Design review of the part shown in the three views and the two pictorial views. Dimensions are in mm from the part's minimum x, y and z. A direction names the side the tool comes from. Coordinates: 2 decimals unless noted, no trailing zeros. Write each loop counter-clockwise with the first axis right and the second up, starting at its lowest first coordinate (ties: lowest second). Pieces come first, ordered by that corner, then holes.
Q1. Take a section at B-B, the plane z = 20. Write out the cut boundary in (x, y), plus the area to 3 significant figures.
Q2. Take a section at A-A, the plane x = 12.5. Write out the cut boundary in (y, z), plus the area to 3 significant figures.
Q3. Take a section at D-D, the plane x = 70. Write out the cut boundary in (y, z), plus the area to 3 significant figures.
Q4. For pin 1 Ø3.5 at (x, y) = (145, 140) entering from +Z; pin 2 Ø8 at (y, z) = (87, 11) entering from -X; pin 3 Ø3 at (y, z) = (141.5, 21.5) entering from +X, all flat-tipped, find the tip position at first contact; note any pin that passes through.
Q5. For L1, parallel to Y at x = 5, z = 3.5; L2, parallel to Y at x = 62.5, z = 21.5; L3, parallel to Y at x = 39, z = 21.75, list the stretches that pass through material, from the lowest coordinate up.
Q6. Take a section at C-C, the plane y = 105. Write out the cut boundary in (x, z), plus the area to 4 significant figures.
Q7. The part is to be moulded in two halves that separate along Y. For the marked faces 3, 4 and 5, say which applies: released by +Y, released by -Y, zero draft, split by the parting line, or undercut.
Q8. For the marked faces 1 and 2, list the 3-axis set-ups (+Z, -Z, +X, -X, +Y, -Y) from which the entire face can be reached by the end or side of a thin tool; tool diameter is ignored.
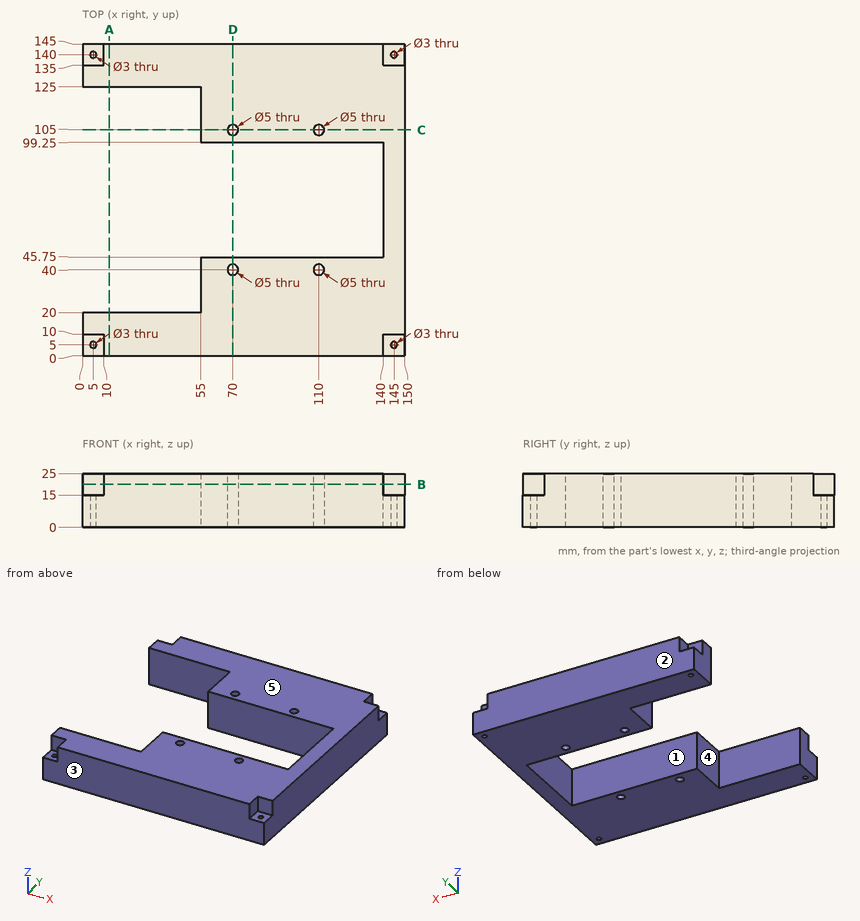
Responses:
1. outline: (0, 10) - (10, 10) - (10, 0) - (140, 0) - (140, 10) - (150, 10) - (150, 135) - (140, 135) - (140, 145) - (10, 145) - (10, 135) - (0, 135) - (0, 125) - (55, 125) - (55, 99.25) - (140, 99.25) - (140, 45.75) - (55, 45.75) - (55, 20) - (0, 20) - close; hole circle Ø5 at (70, 40); hole circle Ø5 at (70, 105); hole circle Ø5 at (110, 40); hole circle Ø5 at (110, 105)
1. area: 10,900 mm2
2. outline: (0, 0) - (20, 0) - (20, 25) - (0, 25) - close; (125, 0) - (145, 0) - (145, 25) - (125, 25) - close
2. area: 1,000 mm2
3. outline: (0, 0) - (37.5, 0) - (37.5, 25) - (0, 25) - close; (42.5, 0) - (45.75, 0) - (45.75, 25) - (42.5, 25) - close; (99.25, 0) - (102.5, 0) - (102.5, 25) - (99.25, 25) - close; (107.5, 0) - (145, 0) - (145, 25) - (107.5, 25) - close
3. area: 2,040 mm2
4. pin 1: stops at z = 15
4. pin 2: stops at x = 140
4. pin 3: stops at x = 140
5. L1: y = 0 to 3.5, 6.5 to 20, 125 to 138.5, 141.5 to 145
5. L2: y = 0 to 45.75, 99.25 to 145
5. L3: y = 0 to 20, 125 to 145
6. outline: (55, 0) - (67.5, 0) - (67.5, 25) - (55, 25) - close; (72.5, 0) - (107.5, 0) - (107.5, 25) - (72.5, 25) - close; (112.5, 0) - (150, 0) - (150, 25) - (112.5, 25) - close
6. area: 2,125 mm2
7. face 3: released by -Y
7. face 4: undercut
7. face 5: zero draft
8. face 1: +Z, -Z, -X
8. face 2: +Z, -Z, +X, -X, +Y
